Verification items for this drawing (mm, ordinates from the low corner). Give positions to 0.01 mm unless a question says otherwise; leave off trailing zeros. Loops run counter-clockwise (first coordinate to the right, second up) from the corner with the lowest first, then second, coordinate; pieces in that order, holes last. Notation, with made-up numbers: (42, -16.75) -> (76, -16.75) arc R36 ccw to (76, 18.25) -> close; hole circle Ø7 at (66.5, 11). An arc over 180 degrees is marked (long way). Answer in a Markdown table with one row per item. Add a question column.
Q1. Section check C-C on x = 224. Enter the section's corners in (y, z) (1 decimal).
Q2. Section check D-D on y = 160. Enter the section's corners in (x, z) (1 decimal), and give its area (3 significant figures).
Q3. Section check B-B on z = 8. Give the number of separate pieces and of enclosed holes in the cut face, and give its area (3 significant figures).
Q4. Section check A-A on y = 127. Enter the section's corners in (x, z) (1 decimal).
Q5. Material ranges on probe 1 along Y at (x, z) = (127, 3.25) (1 decimal); probe 2 along Y at (x, z) = (104, 4.75); probe 3 along Y at (x, z) = (33, 7), recorded low to high.
Q6. Gauge pin test, flat ends, axial feed: P1, Ø6, axis at x = 113.5, z = 6.5, coming from the -Y side (1 decimal); P2, Ø1, axis at x = 87, z = 8.5, coming from the +Y side; P3, Ø2, axis at x = 132.5, z = 2.5, coming from the -Y side; P4, Ø5.5, axis at x = 127, y = 152.4, coming from the -Z side. Record the tip position at first contact, or that the pin passes through.
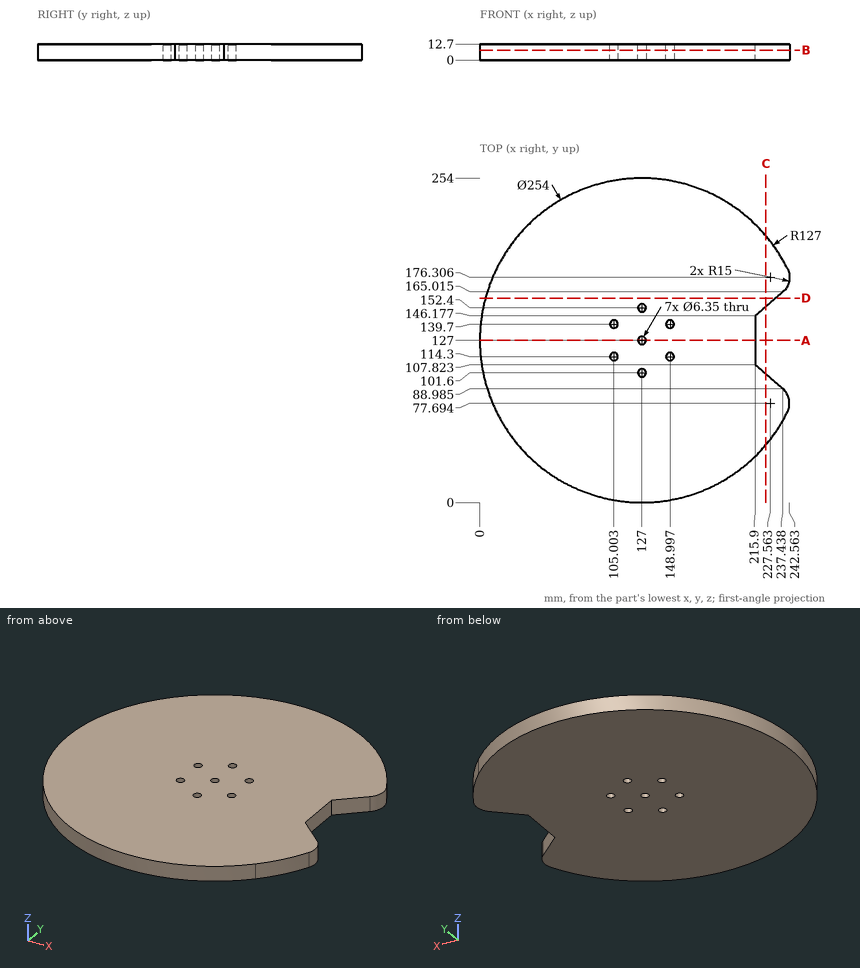
Taken from the geometry:
| question | item | result |
|---|---|---|
| 1 | outline | (45, 0) -> (100.7, 0) -> (100.7, 12.7) -> (45, 12.7) -> close; (153.3, 0) -> (209, 0) -> (209, 12.7) -> (153.3, 12.7) -> close |
| 2 | outline | (4.4, 0) -> (231.7, 0) -> (231.7, 12.7) -> (4.4, 12.7) -> close |
| 2 | area | 2,890 mm² |
| 3 | separate pieces | 1 |
| 3 | enclosed holes | 7 |
| 3 | area | 48,000 mm² |
| 4 | outline | (0, 0) -> (123.8, 0) -> (123.8, 12.7) -> (0, 12.7) -> close; (130.2, 0) -> (215.9, 0) -> (215.9, 12.7) -> (130.2, 12.7) -> close |
| 5 | probe 1 | y = 0 to 98.4, 104.8 to 123.8, 130.2 to 149.2, 155.6 to 254 |
| 5 | probe 2 | y = 2.1 to 111.29, 117.31 to 136.69, 142.71 to 251.9 |
| 5 | probe 3 | y = 41.6 to 212.4 |
| 6 | P1 | stops at y = 0.4 |
| 6 | P2 | stops at y = 247.7 |
| 6 | P3 | stops at y = 0.08 |
| 6 | P4 | passes through |
